Can you work these out from the model? Positions are in its coordinate system, mm. Face numbers are marked on the shaded views. Give positions to 0.01 mm unless a question says otherwise; leave off trailing zeros. Loops run counter-clockwise (first coordinate to the right, second up) from the corner with the lowest first, then second, coordinate; pieces in that order, holes last. Notation, with made-up numbers: (11.5, 46.25) -> (44.5, 46.25) arc R37 cw to (44.5, 82.25) -> close; hole circle Ø2 at (75, -24). An arc over 180 degrees is marked (long way). Return JSON: item names as keys, results as strings. Group by question number.
Q1. Suppose I cut it at A-A, the plane y = 7.75. Please give me the cut outline in (x, z), and give its area (3 significant figures).
Q2. Will these pins go through, and if not, where does the flat tip stop? pin 1 (1 mm diameter, centred on y = 2, z = -4.5, fed in from +X); pin 2 (1.5 mm diameter, centred on y = 10.5, z = 5, fed in from +X); pin 3 (3.5 mm diameter, centred on x = -0.5, z = 0, fed in from +Y).
Q3. I need wall thicknesses on line 1 along Z through (x, y) = (0, 9.65); line 2 along X through (y, z) = (5.5, -1.5); line 3 along X through (y, z) = (11.25, -3.75). Which ranges of each line are inside material? Lowest first, please. Write a range as [from, to].
Q4. Thinking about a two-plate mould opening in Z: for the marked faces 1, 2 and 3, which applies, pulls with the +Z half, pulls with the -Z half, needs draft (parallel to the pull), parting line crosses it, or undercut?
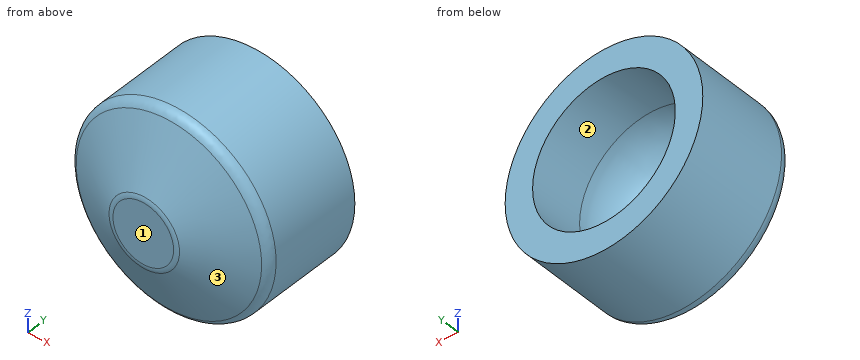
Autodesk Inventor part; units mm, degrees
ref_plane "YZ Plane" through (0, 0, 0) normal (1, 0, 0) x (0, 1, 0)
ref_plane "XZ Plane" through (0, 0, 0) normal (0, 1, 0) x (-1, 0, 0)
ref_plane "XY Plane" through (0, 0, 0) normal (0, 0, 1) x (1, 0, 0)
sketch "Эскиз1" plane through (0, 0, 0) normal (0, 0, 1) x (1, 0, 0)
  line L0 (0, 0) -> (3, 0)
  line L1 (3, 0) -> (9, 3)
  line L2 (9, 3) -> (9, 12)
  line L3 (9, 12) -> (6.5, 12)
  line L4 (6.5, 12) -> (6.5, 7)
  line L5 (0, 2) -> (0, 0)
  line L6 (0, 2) -> (1.5, 2)
  arc A0 (1.5, 2) -> (6.5, 7) centre (1.5, 7) ccw
  dimension "d0" = 18
  dimension "d2" = 13
  dimension "d3" = 12
  dimension "d4" = 9
  dimension "d5" = 6
  dimension "d6" = 10
  dimension "d9" = 1.5
  dimension "d10" = 5
revolve "Вращение1" add sketch "Эскиз1" angle 360 about axis through (0, 2, 0) along (0, -1, 0)
fillet "Сопряжение1" radius 1 2 edges at (-9, 3, 0) (-3, 0, 0)
properties part number "paris_pivot_cup"
Ans:
{
 "1": {"outline": "circle Ø18 at (0, 0); hole circle Ø13 at (0, 0)", "area": "122 mm^2"},
 "2": {"pin 1": "stops at x = 6.66", "pin 2": "stops at x = 7.93", "pin 3": "stops at y = 2.06"},
 "3": {"line 1": "z = [-9, -6.5], [6.5, 9]", "line 2": "x = [-8.87, -6.09], [6.09, 8.87]", "line 3": "x = [-8.18, -5.31], [5.31, 8.18]"},
 "4": {"face 1": "needs draft", "face 2": "undercut", "face 3": "parting line crosses it"}
}
